Can you work these out from the model? Positions are in its coordinate system, mm. Face numbers are marked on the shaded views. A direction names the side the tool comes from. Give positions to 0.01 mm unless a question says otherwise; leave off trailing zeros. Order: outer loops, then holes, each group sorted by start corner. A loop starts at its lowest first (then second) coordinate and runs counter-clockwise, first axis right, second up. Notation, with made-up numbers: M -29.75,13.25 L 28.25,13.25 A28 ccw 28.25,37.25 Z; hole C 80,23 d1. An arc over 180 degrees is marked long. One line per question, with ' | ' between items. Start each with the question number.
1) Please list where these lines run through material, in increasing order: line 1 along X through (y, z) = (2, 20); line 2 along Z through (x, y) = (-4, 4.75); line 3 along X through (y, z) = (4, 1). Write a range as [from, to].
2) If we section it at C-C, the plane x = -30: Please give me the cut outline in (y, z).
3) If we section it at B-B, the plane z = 6: Please give me the cut outline in (x, y).
4) If we section it at A-A, the plane z = -20: Please give me the cut outline in (x, y), plus the area to 3 significant figures.
5) Thinking about a two-plate mould opening in Z: for the marked faces 3, 4 and 5, which applies, +Z half, -Z half, draft (parallel to the pull), parting line (faces both ways), or undercut?
6) If we section it at D-D, the plane y = 2.75: Please give me the cut outline in (x, z), plus the area to 3 significant figures.
7) For the marked faces 1 and 2, which set-ups out of +Z, -Z, +X, -X, +Y, -Y let a thin tool reach every point of the face, with its end or its side?
8) I'm going to push a flat-ended pin straight in: pin 1 Ø4.5 at (x, z) = (-30, 20) entering from +Y. Where does the tip first touch, or does it pass through?
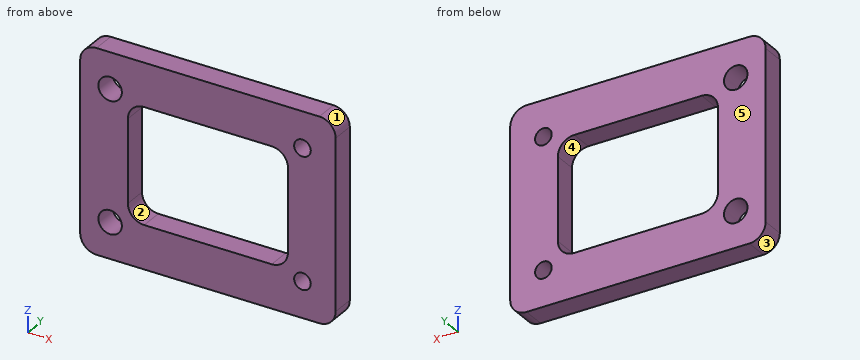
```python
from build123d import *

# Parameters (mm, degrees)
SKETCH1_W           = 78.3542787
SKETCH1_H           = 62.038678242
SKETCH1_R           = 2.55
SKETCH1_R_2         = 3.6
SKETCH1_W_2         = 49.11576042
SKETCH1_H_2         = 35.409761762
BOSS_EXTRUDE1_DEPTH = 7
FILLET2_R           = 5


with BuildPart() as part:
    # Sketch1 → Boss-Extrude1 (new body)
    with BuildSketch(Plane(origin=(0, 0, 0), x_dir=(1, 0, 0), z_dir=(0, 1, 0))):
        Rectangle(SKETCH1_W, SKETCH1_H)
        with Locations(Location((29, 20, 0), (0, 0, 270))):
            Circle(SKETCH1_R, mode=Mode.SUBTRACT)
        with Locations(Location((29, -20, 0), (0, 0, 270))):
            Circle(SKETCH1_R, mode=Mode.SUBTRACT)
        with Locations(Location((-30, -20, 0), (0, 0, 270))):
            Circle(SKETCH1_R_2, mode=Mode.SUBTRACT)
        with Locations(Location((-30, 20, 0), (0, 0, 270))):
            Circle(SKETCH1_R_2, mode=Mode.SUBTRACT)
        Rectangle(SKETCH1_W_2, SKETCH1_H_2, mode=Mode.SUBTRACT)
    extrude(amount=BOSS_EXTRUDE1_DEPTH)

    # Fillet2
    fillet2_edges = [part.edges().sort_by_distance(p)[0] for p in [
        (24.55788021, 3.5, 17.704880881),
        (24.55788021, 3.5, -17.704880881),
        (-24.55788021, 3.5, -17.704880881),
        (-24.55788021, 3.5, 17.704880881),
        (39.17713935, 3.5, 31.019339121),
        (-39.17713935, 3.5, 31.019339121),
        (-39.17713935, 3.5, -31.019339121),
        (39.17713935, 3.5, -31.019339121),
    ]]
    fillet(fillet2_edges, radius=FILLET2_R)


solid = part.part
```
Results found:
1) line 1: x = [-39.18, -33.6], [-26.4, 26.45], [31.55, 39.18] | line 2: z = [-31.02, -17.7], [17.7, 31.02] | line 3: x = [-39.18, -24.56], [24.56, 39.18]
2) outline: M 0,-31.02 L 7,-31.02 L 7,-23.6 L 0,-23.6 Z; M 0,-16.4 L 7,-16.4 L 7,16.4 L 0,16.4 Z; M 0,23.6 L 7,23.6 L 7,31.02 L 0,31.02 Z
3) outline: M -39.18,0 L -24.56,0 L -24.56,7 L -39.18,7 Z; M 24.56,0 L 39.18,0 L 39.18,7 L 24.56,7 Z
4) outline: M -39.18,0 L -33.6,0 L -33.6,7 L -39.18,7 Z; M -26.4,0 L 26.45,0 L 26.45,7 L -26.4,7 Z; M 31.55,0 L 39.18,0 L 39.18,7 L 31.55,7 Z | area: 462 mm²
5) face 3: -Z half | face 4: undercut | face 5: draft
6) outline: M -39.18,-26.02 A5 ccw -34.18,-31.02 L 34.18,-31.02 A5 ccw 39.18,-26.02 L 39.18,26.02 A5 ccw 34.18,31.02 L -34.18,31.02 A5 ccw -39.18,26.02 Z; hole C -30,-20 d7.2; hole C -30,20 d7.2; hole M -24.56,-12.7 A5 ccw -19.56,-17.7 L 19.56,-17.7 A5 ccw 24.56,-12.7 L 24.56,12.7 A5 ccw 19.56,17.7 L -19.56,17.7 A5 ccw -24.56,12.7 Z; hole C 29,-20 d5.1; hole C 29,20 d5.1 | area: 3,000 mm²
7) face 1: +Z, +X, +Y, -Y | face 2: +Y, -Y
8) pin 1: passes through
